```python
from build123d import *

# Parameters (mm, degrees)
SKETCH_1_R          = 1.55
SKETCH_1_W          = 2.95
SKETCH_1_H          = 15
EXTRUDE_1_DEPTH     = 1.5
FILLET_1_R          = 1
SKETCH_2_R          = 0.75
CUT_EXTRUDE_1_DEPTH = 4
CUT_EXTRUDE_2_DEPTH = 4
SKETCH_4_R          = 0.75
CUT_EXTRUDE_3_DEPTH = 4
FILLET_2_R          = 1


with BuildPart() as part:
    # 草图1 → 凸台-拉伸1 (new body, symmetric)
    with BuildSketch(Plane.XY):
        with BuildLine():
            Line((-2.449489743, 12.5), (-11.475, 12.5))
            Line((-11.475, 12.5), (-11.475, -12.5))
            Line((-11.475, -12.5), (-2.449489743, -12.5))
            ThreePointArc((-2.449489743, -12.5), (1.355873501, -13.226702194), (3.5, -10))
            Line((3.5, -10), (3.5, 10))
            ThreePointArc((3.5, 10), (1.355873501, 13.226702194), (-2.449489743, 12.5))
        make_face()
        with Locations((0, 10)):
            Circle(SKETCH_1_R, mode=Mode.SUBTRACT)
        with Locations((0, -10)):
            Circle(SKETCH_1_R, mode=Mode.SUBTRACT)
        with Locations((-6.5, 0)):
            Rectangle(SKETCH_1_W, SKETCH_1_H, mode=Mode.SUBTRACT)
    extrude(amount=EXTRUDE_1_DEPTH, both=True)

    # 圆角1
    fillet_1_edges = [part.edges().sort_by_distance(p)[0] for p in [
        (-11.475, -12.5, 0),
        (-11.475, 12.5, 0),
    ]]
    fillet(fillet_1_edges, radius=FILLET_1_R)

    # 草图2 → 切除-拉伸1 (cut, through all)
    with BuildSketch(Plane.XY.offset(1.5)):
        with Locations((-7.975, 6.75)):
            Circle(SKETCH_2_R)
        with Locations((-5.025, 6.75)):
            Circle(SKETCH_2_R)
        with Locations((-7.975, -6.75)):
            Circle(SKETCH_2_R)
        with Locations((-5.025, -6.75)):
            Circle(SKETCH_2_R)
    extrude(amount=-CUT_EXTRUDE_1_DEPTH, mode=Mode.SUBTRACT)

    # 草图3 → 切除-拉伸2 (cut, through all)
    with BuildSketch(Plane.XY.offset(1.5)):
        Polygon((3.5, 8.5), (0, 5.166666667), (0, -5.166666667), (3.5, -8.5), align=None)
    extrude(amount=-CUT_EXTRUDE_2_DEPTH, mode=Mode.SUBTRACT)

    # 草图4 → 切除-拉伸3 (cut, through all)
    with BuildSketch(Plane.XY.offset(1.5)):
        with Locations((0, 4.416666667)):
            Circle(SKETCH_4_R)
        with Locations((0, -4.416666667)):
            Circle(SKETCH_4_R)
    extrude(amount=-CUT_EXTRUDE_3_DEPTH, mode=Mode.SUBTRACT)

    # 圆角2
    fillet_2_edges = [part.edges().sort_by_distance(p)[0] for p in [
        (-2.449489743, 12.5, 0),
        (-2.449489743, -12.5, 0),
        (3.5, 8.5, 0),
        (3.5, -8.5, 0),
    ]]
    fillet(fillet_2_edges, radius=FILLET_2_R)


solid = part.part
```
Design review of the part built by this model. Coordinates are the model's own, in mm. A direction names the side the tool comes from. Coordinates: 2 decimals unless noted, no trailing zeros. Order: outer loops, then holes, each group sorted by start corner. A loop starts at its lowest first (then second) coordinate and runs counter-clockwise, first axis right, second up. Notation, with made-up numbers: (24.25, -29.75) - (34.25, -29.75) arc R17 cw to (34.25, -24.75) - close; hole circle Ø9 at (84.5, -12). An arc over 180 degrees is marked (long way). One line per question, with ' | ' between items.
Q1. Clearance check with flat-ended pins moving along their axes: pin 1 Ø1.5 at (y, z) = (-0.5, 0.5) entering from +X; pin 2 Ø1.5 at (x, z) = (-6.5, 0) entering from +Y; pin 3 Ø1.5 at (x, z) = (-7, 0.5) entering from -Y. State where each tip first meets the part, or that it passes through.
Answer key:
pin 1: stops at x = 0 | pin 2: stops at y = 12.5 | pin 3: stops at y = -12.5
Q2. For faces 1 (the flat face through (-7, 12.5, 0)), 2 (the flat face through (-7, -12.5, 0)), 3 (the flat face through (1.62, 6.71, 0.02)), list the 3-axis set-ups (+Z, -Z, +X, -X, +Y, -Y) from which the entire face can be reached by the end or side of a thin tool; tool diameter is ignored.
Answer key:
face 1: +Z, -Z, -X, +Y | face 2: +Z, -Z, -X, -Y | face 3: +Z, -Z, +X
Q3. Consider section B-B, the plane z = -1.15. Give the boundary of the cut face in (x, y) (3 decimals), then the cut area to 3 significant figures.
Answer key:
outline: (-11.475, -11.5) arc R1 ccw to (-10.475, -12.5) - (-2.828, -12.5) arc R1 cw to (-2.2, -12.722) arc R3.5 ccw to (3.5, -10) - (3.5, -8.929) arc R1 ccw to (3.19, -8.204) - (0, -5.167) arc R0.75 cw to (0, -3.667) - (0, 3.667) arc R0.75 cw to (0, 5.167) - (3.19, 8.204) arc R1 ccw to (3.5, 8.929) - (3.5, 10) arc R3.5 ccw to (-2.2, 12.722) arc R1 cw to (-2.828, 12.5) - (-10.475, 12.5) arc R1 ccw to (-11.475, 11.5) - close; hole (-7.975, -7.5) - (-5.025, -7.5) arc R0.75 ccw to (-5.025, -6) - (-5.025, 6) arc R0.75 ccw to (-5.025, 7.5) - (-7.975, 7.5) arc R0.75 ccw to (-7.975, 6) - (-7.975, -6) arc R0.75 ccw to start; hole circle Ø3.1 at (0, -10); hole circle Ø3.1 at (0, 10) | area: 267 mm2
Q4. Consider section A-A, the plane y = 5.5. Give the boundary of the cut face in (x, z) (3 decimals).
Answer key:
outline: (-11.475, -1.5) - (-7.975, -1.5) - (-7.975, 1.5) - (-11.475, 1.5) - close; (-5.025, -1.5) - (0.35, -1.5) - (0.35, 1.5) - (-5.025, 1.5) - close
Q5. Consider section D-D, the plane x = -9. Give the boundary of the cut face in (y, z), then the cut area to 3 significant figures.
Answer key:
outline: (-12.5, -1.5) - (12.5, -1.5) - (12.5, 1.5) - (-12.5, 1.5) - close | area: 75.0 mm2
Q6. Consider section C-C, the plane y = -6.75. Give the boundary of the cut face in (x, z) (1 decimal).
Answer key:
outline: (-11.5, -1.5) - (-8.7, -1.5) - (-8.7, 1.5) - (-11.5, 1.5) - close; (-4.3, -1.5) - (1.7, -1.5) - (1.7, 1.5) - (-4.3, 1.5) - close
Q7. The part is to be moulded in two halves that separate along X. For faces 4 (the cylindrical face through (-0.75, -4.4, 0.02)), 5 (the flat face through (-7, 7.5, 0)), 6 (the flat face through (-11.475, 0, 0)), say which applies: +X half, -X half, draft (parallel to the pull), parting line (faces both ways), or undercut.
Answer key:
face 4: +X half | face 5: undercut | face 6: -X half
Q8. To check wall thickness, follow line 1 along X through (y, z) = (-1.5, 0.45) (3 decimals); line 2 along Y through (x, z) = (-0.25, -1.2); line 3 along Y through (x, z) = (-1, -0.45). State the ranges of each line that lie inside material, in increasing order.
Answer key:
line 1: x = -11.475 to -7.975, -5.025 to 0 | line 2: y = -13.49 to -11.53, -8.47 to -5.12, -3.71 to 3.71, 5.12 to 8.47, 11.53 to 13.49 | line 3: y = -13.35 to -11.18, -8.82 to 8.82, 11.18 to 13.35
